from build123d import *

# Parameters (mm, degrees)
RESSALTO_EXTRUS_O4_DEPTH = 8
ESBO_O7_R                = 4.1
CORTE_EXTRUS_O3_DEPTH    = 8
ESBO_O8_R                = 8
ESBO_O8_R_2              = 4.1
RESSALTO_EXTRUS_O5_DEPTH = 6
ESBO_O14_R               = 5.515467334
ESBO_O14_R_2             = 4.1
RESSALTO_EXTRUS_O8_DEPTH = 8
FILETE3_R                = 15
CORTE_EXTRUS_O6_DEPTH    = 8


with BuildPart() as part:
    # Esboço1 → Ressalto-extrusão4 (new body)
    with BuildSketch(Plane(origin=(0, 0, 0), x_dir=(1, 0, 0), z_dir=(0, 1, 0))):
        with BuildLine():
            Line((-8.455093814, 52.012944842), (6.19830879, 52.012944842))
            Line((6.19830879, 52.012944842), (6.19830879, 57.528412176))
            Line((6.19830879, 57.528412176), (-8.455093814, 57.528412176))
            add(Edge.make_bspline(
                [(-40, 15), (-41.806500993, 47.170631402), (-8.455093814, 57.528412176)],
                knots=[0, 0, 0, 1, 1, 1], degree=2))
            Line((-40, 15), (-40, 0))
            Line((-40, 0), (-34, 0))
            Line((-34, 0), (-34, 15))
            add(Edge.make_bspline(
                [(-34, 15), (-35.042952492, 42.040177947), (-8.455093814, 52.012944842)],
                knots=[0, 0, 0, 1, 1, 1], degree=2))
        make_face()
    extrude(amount=RESSALTO_EXTRUS_O4_DEPTH)

    # Esboço7 → Corte-extrusão3 (cut)
    with BuildSketch(Plane(origin=(-34, 0, 0), x_dir=(0, 0, -1), z_dir=(1, 0, 0))):
        with Locations((0, 8)):
            Circle(ESBO_O7_R)
    extrude(amount=-CORTE_EXTRUS_O3_DEPTH, mode=Mode.SUBTRACT)

    # Esboço8 → Ressalto-extrusão5 (add)
    with BuildSketch(Plane(origin=(-34, 0, 0), x_dir=(0, 0, -1), z_dir=(1, 0, 0))):
        with Locations((0, 8)):
            Circle(ESBO_O8_R)
        with Locations((0, 8)):
            Circle(ESBO_O8_R_2, mode=Mode.SUBTRACT)
    extrude(amount=-RESSALTO_EXTRUS_O5_DEPTH)

    # Esboço14 → Ressalto-extrusão8 (add)
    with BuildSketch(Plane(origin=(0, 8, 0), x_dir=(1, 0, 0), z_dir=(0, 1, 0))):
        with Locations((6.19830879, 57.528412176)):
            Circle(ESBO_O14_R)
        with Locations((6.19830879, 57.528412176)):
            Circle(ESBO_O14_R_2, mode=Mode.SUBTRACT)
    extrude(amount=-RESSALTO_EXTRUS_O8_DEPTH)

    # Filete3
    filete3_edges = [part.edges().sort_by_distance(p)[0] for p in [
        (0.682841456, 4, -57.528412176),
    ]]
    fillet(filete3_edges, radius=FILETE3_R)

    # Esboço15 → Corte-extrusão6 (cut)
    with BuildSketch(Plane(origin=(0, 8, 0), x_dir=(1, 0, 0), z_dir=(0, 1, 0))):
        with BuildLine():
            Line((6.19830879, 57.528412176), (2.09830879, 57.528412176))
            ThreePointArc((2.09830879, 57.528412176), (3.299170987, 54.629274373), (6.19830879, 53.428412176))
            Line((6.19830879, 53.428412176), (6.19830879, 57.528412176))
        make_face()
    extrude(amount=-CORTE_EXTRUS_O6_DEPTH, mode=Mode.SUBTRACT)


solid = part.part
Source: CAD feature listing. Evaluate the final solid. Frame: model axes, mm. A direction names the side the tool comes from. Coordinates: 2 decimals unless noted, no trailing zeros. Order: outer loops, then holes, each group sorted by start corner. A loop starts at its lowest first (then second) coordinate and runs counter-clockwise, first axis right, second up. Notation, with made-up numbers: M 58.5,-22.5 L 109.5,-22.5 A15 ccw 109.5,-9.5 Z; hole C 64,12 d5. An arc over 180 degrees is marked long. Write each question's results on one line, items separated by ' | '. Start each with the question number.
1. Section B-B, the plane y = 11. Return the cut outline in (x, z).
2. Material intervals for L1, parallel to Y at x = -36, z = 0; L2, parallel to X at y = 14.5, z = 1; L3, parallel to Z at x = -37.5, y = 12.5, sorted ascending.
3. Pin query (flat end, axial travel): pin 1 (3 mm diameter, centred on y = 10.5, z = -6.5, fed in from +X); pin 2 (3 mm diameter, centred on x = -35, y = 7, fed in from -Z); pin 3 (15.5 mm diameter, centred on x = -15, z = -45, fed in from +Y). Return the tip coordinate at first contact, or that it passes through.
4. Section C-C, the plane z = -7. Return the cut outline in (x, y), then the cut area to 3 significant figures.
5. Section D-D, the plane x = -4. Return the cut outline in (y, z).
6. Section A-A, the plane x = 7. Return the cut outline in (y, z).
7. Draft query along Z for faces 4 (the face through (-37, 4, 0.9)), 5 (the face through (-2.225, 4.056, -58.602)), 6 (the face through (-40, 4.6, -3.3)). Return one class per face: +Z half, -Z half, draft (parallel to the pull), parting line (faces both ways), or undercut.
8. Reachability of faces 1 (the face through (-36.96, 13.84, 5.47)), 2 (the face through (-1, 4, -52.013)), 3 (the face through (-27, 8, -42)) from +Z, -Z, +X, -X, +Y, -Y: full face, straight path, thin tool, end or side. Return the list, or none.
Solution:
1) outline: M -40,-7.42 L -34,-7.42 L -34,-2.79 L -40,-2.79 Z; M -40,2.79 L -34,2.79 L -34,7.42 L -40,7.42 Z
2) L1: 0 to 3.9, 12.1 to 16 | L2: -40 to -34 | L3: -6.61 to 6.61
3) pin 1: x = -34 | pin 2: z = -41.05 | pin 3: y = 8
4) outline: M -40,0 L -34,0 L -34,11.87 L -40,11.87 Z | area: 71.2 mm²
5) outline: M 0,-58.02 L 8,-58.02 L 8,-52.01 L 0,-52.01 Z
6) outline: M 0,-62.99 L 8,-62.99 L 8,-61.55 L 0,-61.55 Z; M 0,-53.51 L 8,-53.51 L 8,-52.07 L 0,-52.07 Z
7) face 4: undercut | face 5: -Z half | face 6: draft
8) face 1: +X, -X | face 2: +Z, +X, +Y, -Y | face 3: -Z, +X, -X, +Y
